```python
from build123d import *

# Parameters (mm, degrees)
SKETCH1_W           = 8
SKETCH1_H           = 8
BOSS_EXTRUDE1_DEPTH = 20
CUT_EXTRUDE1_DEPTH  = 20
CUT_EXTRUDE8_DEPTH  = 4
FILLET1_R           = 1
FILLET2_R           = 1


with BuildPart() as part:
    # Sketch1 → Boss-Extrude1 (new body)
    with BuildSketch(Plane.XY):
        with Locations((1.399149149, 0.658917954)):
            Rectangle(SKETCH1_W, SKETCH1_H)
    extrude(amount=BOSS_EXTRUDE1_DEPTH)

    # Sketch4 → Cut-Extrude1 (cut)
    with BuildSketch(Plane.XY.offset(20)):
        with BuildLine():
            ThreePointArc((3.399149149, 0.658917954), (2.164516014, 2.506677019), (-0.015064413, 2.073131517))
            Line((-0.015064413, 2.073131517), (2.813362712, -0.755295608))
            ThreePointArc((2.813362712, -0.755295608), (3.246908214, -0.10644891), (3.399149149, 0.658917954))
        make_face()
        with BuildLine():
            Line((2.813362712, -0.755295608), (-0.015064413, 2.073131517))
            ThreePointArc((-0.015064413, 2.073131517), (-0.015064413, -0.755295608), (2.813362712, -0.755295608))
        make_face()
    extrude(amount=-CUT_EXTRUDE1_DEPTH, mode=Mode.SUBTRACT)

    # Sketch5 → Cut-Extrude8 (cut)
    with BuildSketch(Plane.XY.offset(20)):
        Polygon((-2.500850851, 0.658917954), (-0.550850851, -2.71858112), (3.349149149, -2.71858112), (5.299149149, 0.658917954), (3.349149149, 4.036417029), (-0.550850851, 4.036417029), align=None)
    extrude(amount=-CUT_EXTRUDE8_DEPTH, mode=Mode.SUBTRACT)

    # Fillet1
    fillet1_edges = [part.edges().sort_by_distance(p)[0] for p in [
        (-2.600850851, 4.658917954, 10),
        (5.399149149, 4.658917954, 10),
        (5.399149149, -3.341082046, 10),
    ]]
    fillet(fillet1_edges, radius=FILLET1_R)

    # Fillet2
    fillet2_edges = [part.edges().sort_by_distance(p)[0] for p in [
        (-2.600850851, -3.341082046, 10),
    ]]
    fillet(fillet2_edges, radius=FILLET2_R)


solid = part.part
```
CAD build for the part. Positions are in the model's coordinates, mm. A direction names the side the tool comes from. Give positions to 0.01 mm unless a question says otherwise; leave off trailing zeros. Write each loop counter-clockwise with the first axis right and the second up, starting at its lowest first coordinate (ties: lowest second). Pieces come first, ordered by that corner, then holes. Notation, with made-up numbers: M -37.5,-28 L -11.5,-28 A22 cw -11.5,-1 Z; hole C 16,-31 d9. An arc over 180 degrees is marked long. Return JSON: item names as keys, results as strings. Group by question number.
(1) Drill centre lines: L1, parallel to Y at x = 1.25, z = 16.75; L2, parallel to X at y = 0.5, z = 3; L3, parallel to Z at x = 0, y = -2. Where is each one in solid material? Low to high. Write a range as [from, to].
(2) 3-axis set-ups, long thin cutter, end or side, ignore diameter. For faces 4 (the face through (5.1, 4.37, 10.14)), 5 (the face through (4.31, -1.053, 18.028)): which of +Z, -Z, +X, -X, +Y, -Y reach the whole face in a straight line?
(3) Flat gauge pin, fed straight in: pin 1 Ø1.5 at (x, y) = (4, 0) entering from +Z. Where does the tip first touch, or does it go through?
(4) Band-saw the part on C-C (y = 0). Give the cut face in (x, z).
(5) Band-saw the part on A-A (x = 0.5). Give the cut face in (y, z), and give its area (3 significant figures).
(6) Mould opens along X. For faces 1 (the face through (1, -3, 20)), 2 (the face through (-2.316, -3.04, 10.14)), 3 (the face through (-1.54, -1.006, 18.028)) say: pulls with the +X half, pulls with the -X half, needs draft (parallel to the pull), parting line crosses it, or undercut.
(7) Band-saw the part on D-D (y = 3). Give the cut face in (x, z), and give its area (3 significant figures).
(8) Band-saw the part on B-B (z = 6). Give the cut face in (x, y).
Entries:
{
 "1": {"L1": "y = [-3.34, -2.72], [4.04, 4.66]", "L2": "x = [-2.6, -0.59], [3.39, 5.4]", "L3": "z = [0, 16]"},
 "2": {"face 4": "+Z, -Z, +X, +Y", "face 5": "+Z"},
 "3": {"pin 1": "stops at z = 16"},
 "4": {"outline": "M -2.6,0 L -0.49,0 L -0.49,16 L -2.12,16 L -2.12,20 L -2.6,20 Z; M 3.29,0 L 5.4,0 L 5.4,20 L 4.92,20 L 4.92,16 L 3.29,16 Z"},
 "5": {"outline": "M -3.34,0 L -1.13,0 L -1.13,16 L -2.72,16 L -2.72,20 L -3.34,20 Z; M 2.45,0 L 4.66,0 L 4.66,20 L 4.04,20 L 4.04,16 L 2.45,16 Z", "area": "75.8 mm^2"},
 "6": {"face 1": "needs draft", "face 2": "pulls with the -X half", "face 3": "undercut"},
 "7": {"outline": "M -2.6,0 L 5.4,0 L 5.4,20 L 3.95,20 L 3.95,16 L -1.15,16 L -1.15,20 L -2.6,20 Z", "area": "140 mm^2"},
 "8": {"outline": "M -2.6,-2.34 A1 ccw -1.6,-3.34 L 4.4,-3.34 A1 ccw 5.4,-2.34 L 5.4,3.66 A1 ccw 4.4,4.66 L -1.6,4.66 A1 ccw -2.6,3.66 Z; hole C 1.4,0.66 d4"}
}
